Verification items for the finished model (mm, model axes). A direction names the side the tool comes from. Coordinates: 2 decimals unless noted, no trailing zeros. Write each loop counter-clockwise with the first axis right and the second up, starting at its lowest first coordinate (ties: lowest second). Pieces come first, ordered by that corner, then holes. Notation, with made-up numbers: M 10.25,69 L 24.25,69 A17 ccw 24.25,81 Z; hole C 82,51.25 d7. An arc over 180 degrees is marked long. Answer in a Markdown table with one row per item.
from build123d import *

# Parameters (mm, degrees)
BOX024_W                  = 130
BOX024_H                  = 2
BOX024_DEPTH              = 2
BOX025_W                  = 79
BOX025_H                  = 2
BOX025_DEPTH              = 2
BOX026_W                  = 2
BOX026_H                  = 52
BOX026_DEPTH              = 2
BOX023_W                  = 2
BOX023_H                  = 53
BOX023_DEPTH              = 2
BOX018_W                  = 0.5
BOX018_H                  = 2
BOX018_DEPTH              = 12
BOX019_W                  = 0.5
BOX019_H                  = 2
BOX019_DEPTH              = 12
BOX020_W                  = 0.5
BOX020_H                  = 2
BOX020_DEPTH              = 12
BOX021_W                  = 0.5
BOX021_H                  = 2
BOX021_DEPTH              = 12
BOX022_W                  = 0.5
BOX022_H                  = 2
BOX022_DEPTH              = 12
BOX017_W                  = 0.5
BOX017_H                  = 2
BOX017_DEPTH              = 12
BOX015_W                  = 12
BOX015_H                  = 10
BOX015_DEPTH              = 20
BOX016_W                  = 12
BOX016_H                  = 10
BOX016_DEPTH              = 20
BOX014_W                  = 12
BOX014_H                  = 10
BOX014_DEPTH              = 20
CYLINDER016_R             = 7
CYLINDER016_DEPTH         = 1.5
CYLINDER015_R             = 6
CYLINDER015_DEPTH         = 18
FUSION006_PLACEMENT_ANGLE = 90
CYLINDER018_R             = 7
CYLINDER018_DEPTH         = 1.5
CYLINDER017_R             = 6
CYLINDER017_DEPTH         = 18
FUSION007_PLACEMENT_ANGLE = 90
CYLINDER014_R             = 7
CYLINDER014_DEPTH         = 1.5
CYLINDER013_R             = 6
CYLINDER013_DEPTH         = 18
FUSION005_PLACEMENT_ANGLE = 90
BOX013_W                  = 33
BOX013_H                  = 77
BOX013_DEPTH              = 17
BOX012_W                  = 10
BOX012_H                  = 11
BOX012_DEPTH              = 21
BOX011_W                  = 13.5
BOX011_H                  = 11
BOX011_DEPTH              = 21
CYLINDER010_R             = 3.1
CYLINDER010_DEPTH         = 20
CYLINDER011_R             = 3.1
CYLINDER011_DEPTH         = 20
CYLINDER012_R             = 3.1
CYLINDER012_DEPTH         = 20
BOX004_W                  = 20
BOX004_H                  = 67
BOX004_DEPTH              = 20
BOX005_W                  = 20
BOX005_H                  = 67
BOX005_DEPTH              = 20
BOX006_W                  = 20
BOX006_H                  = 67
BOX006_DEPTH              = 20
BOX007_W                  = 14
BOX007_H                  = 40
BOX007_DEPTH              = 20
BOX008_W                  = 54
BOX008_H                  = 69
BOX008_DEPTH              = 20
BOX009_W                  = 30
BOX009_H                  = 52
BOX009_DEPTH              = 20
BOX010_W                  = 72
BOX010_H                  = 52
BOX010_DEPTH              = 6
CYLINDER009_R             = 3.1
CYLINDER009_DEPTH         = 20
BOX_W                     = 192
BOX_H                     = 81
BOX_DEPTH                 = 22
FILLET_R                  = 3


with BuildPart() as cube011:
    # Box024 → Box024 (new body)
    with BuildSketch(Plane(origin=(12, 75, 21), x_dir=(1, 0, 0), z_dir=(0, 0, 1))):
        with Locations((65, 1)):
            Rectangle(BOX024_W, BOX024_H)
    extrude(amount=BOX024_DEPTH)


with BuildPart() as cube012:
    # Box025 → Box025 (new body)
    with BuildSketch(Plane(origin=(12, 4, 21), x_dir=(1, 0, 0), z_dir=(0, 0, 1))):
        with Locations((39.5, 1)):
            Rectangle(BOX025_W, BOX025_H)
    extrude(amount=BOX025_DEPTH)


with BuildPart() as cube013:
    # Box026 → Box026 (new body)
    with BuildSketch(Plane(origin=(186, 14, 21), x_dir=(1, 0, 0), z_dir=(0, 0, 1))):
        with Locations((1, 26)):
            Rectangle(BOX026_W, BOX026_H)
    extrude(amount=BOX026_DEPTH)


with BuildPart() as latches:
    # Box023 → Box023 (new body)
    with BuildSketch(Plane(origin=(2, 14, 21), x_dir=(1, 0, 0), z_dir=(0, 0, 1))):
        with Locations((1, 26.5)):
            Rectangle(BOX023_W, BOX023_H)
    extrude(amount=BOX023_DEPTH)

    # Compound: union Cube011, Cube012, Cube013
    add(cube011.part)
    add(cube012.part)
    add(cube013.part)


with BuildPart() as cube005:
    # Box018 → Box018 (new body)
    with BuildSketch(Plane(origin=(163.5, 0, 9), x_dir=(1, 0, 0), z_dir=(0, 0, 1))):
        with Locations((0.25, 1)):
            Rectangle(BOX018_W, BOX018_H)
    extrude(amount=BOX018_DEPTH)


with BuildPart() as cube006:
    # Box019 → Box019 (new body)
    with BuildSketch(Plane(origin=(167.5, 0, 9), x_dir=(1, 0, 0), z_dir=(0, 0, 1))):
        with Locations((0.25, 1)):
            Rectangle(BOX019_W, BOX019_H)
    extrude(amount=BOX019_DEPTH)


with BuildPart() as cube007:
    # Box020 → Box020 (new body)
    with BuildSketch(Plane(origin=(179, 0, 9), x_dir=(1, 0, 0), z_dir=(0, 0, 1))):
        with Locations((0.25, 1)):
            Rectangle(BOX020_W, BOX020_H)
    extrude(amount=BOX020_DEPTH)


with BuildPart() as cube008:
    # Box021 → Box021 (new body)
    with BuildSketch(Plane(origin=(175.5, 79, 9), x_dir=(1, 0, 0), z_dir=(0, 0, 1))):
        with Locations((0.25, 1)):
            Rectangle(BOX021_W, BOX021_H)
    extrude(amount=BOX021_DEPTH)


with BuildPart() as cube009:
    # Box022 → Box022 (new body)
    with BuildSketch(Plane(origin=(164, 79, 9), x_dir=(1, 0, 0), z_dir=(0, 0, 1))):
        with Locations((0.25, 1)):
            Rectangle(BOX022_W, BOX022_H)
    extrude(amount=BOX022_DEPTH)


with BuildPart() as obj1:
    # Box017 → Box017 (new body)
    with BuildSketch(Plane(origin=(152, 0, 9), x_dir=(1, 0, 0), z_dir=(0, 0, 1))):
        with Locations((0.25, 1)):
            Rectangle(BOX017_W, BOX017_H)
    extrude(amount=BOX017_DEPTH)

    # Fusion010: union Cube005, Cube006, Cube007, Cube008, Cube009
    add(cube005.part)
    add(cube006.part)
    add(cube007.part)
    add(cube008.part)
    add(cube009.part)


with BuildPart() as cube002:
    # Box015 → Box015 (new body)
    with BuildSketch(Plane(origin=(167.5, 0, 13), x_dir=(1, 0, 0), z_dir=(0, 0, 1))):
        with Locations((6, 5)):
            Rectangle(BOX015_W, BOX015_H)
    extrude(amount=BOX015_DEPTH)


with BuildPart() as cube003:
    # Box016 → Box016 (new body)
    with BuildSketch(Plane(origin=(164, 71, 13), x_dir=(1, 0, 0), z_dir=(0, 0, 1))):
        with Locations((6, 5)):
            Rectangle(BOX016_W, BOX016_H)
    extrude(amount=BOX016_DEPTH)


with BuildPart() as fusion009:
    # Box014 → Box014 (new body)
    with BuildSketch(Plane(origin=(152, 0, 13), x_dir=(1, 0, 0), z_dir=(0, 0, 1))):
        with Locations((6, 5)):
            Rectangle(BOX014_W, BOX014_H)
    extrude(amount=BOX014_DEPTH)

    # Fusion009: union Cube002, Cube003
    add(cube002.part)
    add(cube003.part)


with BuildPart() as cylinder016:
    # Cylinder016 → Cylinder016 (new body)
    with BuildSketch(Plane.XY):
        Circle(CYLINDER016_R)
    extrude(amount=CYLINDER016_DEPTH)


with BuildPart() as fusion006:
    # Cylinder015 → Cylinder015 (new body)
    with BuildSketch(Plane.XY):
        Circle(CYLINDER015_R)
    extrude(amount=CYLINDER015_DEPTH)

    # Fusion006: union Cylinder016
    add(cylinder016.part)


with BuildPart() as fusion006_1:
    # Fusion006 placement: moved
    add(fusion006.part.moved(Location((158, -2, 13))).rotate(Axis((158, -2, 13), (-1, 0, 0)), FUSION006_PLACEMENT_ANGLE))


with BuildPart() as cylinder018:
    # Cylinder018 → Cylinder018 (new body)
    with BuildSketch(Plane.XY):
        Circle(CYLINDER018_R)
    extrude(amount=CYLINDER018_DEPTH)


with BuildPart() as fusion007:
    # Cylinder017 → Cylinder017 (new body)
    with BuildSketch(Plane.XY):
        Circle(CYLINDER017_R)
    extrude(amount=CYLINDER017_DEPTH)

    # Fusion007: union Cylinder018
    add(cylinder018.part)


with BuildPart() as fusion007_1:
    # Fusion007 placement: moved
    add(fusion007.part.moved(Location((170, 82.5, 13))).rotate(Axis((170, 82.5, 13), (1, 0, 0)), FUSION007_PLACEMENT_ANGLE))


with BuildPart() as cylinder014:
    # Cylinder014 → Cylinder014 (new body)
    with BuildSketch(Plane.XY):
        Circle(CYLINDER014_R)
    extrude(amount=CYLINDER014_DEPTH)


with BuildPart() as dc_jack_holes:
    # Cylinder013 → Cylinder013 (new body)
    with BuildSketch(Plane.XY):
        Circle(CYLINDER013_R)
    extrude(amount=CYLINDER013_DEPTH)

    # Fusion005: union Cylinder014
    add(cylinder014.part)


with BuildPart() as dc_jack_holes_1:
    # Fusion005 placement: moved
    add(dc_jack_holes.part.moved(Location((173.5, -2, 13))).rotate(Axis((173.5, -2, 13), (-1, 0, 0)), FUSION005_PLACEMENT_ANGLE))

    # Fusion008: union Fusion006, Fusion007
    add(fusion006_1.part)
    add(fusion007_1.part)


with BuildPart() as cube:
    # Box013 → Box013 (new body)
    with BuildSketch(Plane(origin=(149, 2, 4), x_dir=(1, 0, 0), z_dir=(0, 0, 1))):
        with Locations((16.5, 38.5)):
            Rectangle(BOX013_W, BOX013_H)
    extrude(amount=BOX013_DEPTH)


with BuildPart() as obj2:
    # Box012 → Box012 (new body)
    with BuildSketch(Plane(origin=(138.5, -1, 4), x_dir=(1, 0, 0), z_dir=(0, 0, 1))):
        with Locations((5, 5.5)):
            Rectangle(BOX012_W, BOX012_H)
    extrude(amount=BOX012_DEPTH)


with BuildPart() as arduino_jacks_holes:
    # Box011 → Box011 (new body)
    with BuildSketch(Plane(origin=(106.5, -1, 4), x_dir=(1, 0, 0), z_dir=(0, 0, 1))):
        with Locations((6.75, 5.5)):
            Rectangle(BOX011_W, BOX011_H)
    extrude(amount=BOX011_DEPTH)

    # Fusion004: union obj2
    add(obj2.part)


with BuildPart() as m4_mounting_hole001:
    # Cylinder010 → Cylinder010 (new body)
    with BuildSketch(Plane(origin=(2, 77, 1), x_dir=(1, 0, 0), z_dir=(0, 0, 1))):
        Circle(CYLINDER010_R)
    extrude(amount=CYLINDER010_DEPTH)


with BuildPart() as m4_mounting_hole002:
    # Cylinder011 → Cylinder011 (new body)
    with BuildSketch(Plane(origin=(186, 77, 1), x_dir=(1, 0, 0), z_dir=(0, 0, 1))):
        Circle(CYLINDER011_R)
    extrude(amount=CYLINDER011_DEPTH)


with BuildPart() as m4_mounting_hole003:
    # Cylinder012 → Cylinder012 (new body)
    with BuildSketch(Plane(origin=(186, 4, 1), x_dir=(1, 0, 0), z_dir=(0, 0, 1))):
        Circle(CYLINDER012_R)
    extrude(amount=CYLINDER012_DEPTH)


with BuildPart() as obj3:
    # Box004 → Box004 (new body)
    with BuildSketch(Plane(origin=(6, 7, 1), x_dir=(1, 0, 0), z_dir=(0, 0, 1))):
        with Locations((10, 33.5)):
            Rectangle(BOX004_W, BOX004_H)
    extrude(amount=BOX004_DEPTH)


with BuildPart() as obj4:
    # Box005 → Box005 (new body)
    with BuildSketch(Plane(origin=(29, 7, 1), x_dir=(1, 0, 0), z_dir=(0, 0, 1))):
        with Locations((10, 33.5)):
            Rectangle(BOX005_W, BOX005_H)
    extrude(amount=BOX005_DEPTH)


with BuildPart() as obj5:
    # Box006 → Box006 (new body)
    with BuildSketch(Plane(origin=(52, 7, 1), x_dir=(1, 0, 0), z_dir=(0, 0, 1))):
        with Locations((10, 33.5)):
            Rectangle(BOX006_W, BOX006_H)
    extrude(amount=BOX006_DEPTH)


with BuildPart() as obj6:
    # Box007 → Box007 (new body)
    with BuildSketch(Plane(origin=(74, 18, 1), x_dir=(1, 0, 0), z_dir=(0, 0, 1))):
        with Locations((7, 20)):
            Rectangle(BOX007_W, BOX007_H)
    extrude(amount=BOX007_DEPTH)


with BuildPart() as obj7:
    # Box008 → Box008 (new body)
    with BuildSketch(Plane(origin=(98, 2, 1), x_dir=(1, 0, 0), z_dir=(0, 0, 1))):
        with Locations((27, 34.5)):
            Rectangle(BOX008_W, BOX008_H)
    extrude(amount=BOX008_DEPTH)


with BuildPart() as obj8:
    # Box009 → Box009 (new body)
    with BuildSketch(Plane(origin=(156, 14, 1), x_dir=(1, 0, 0), z_dir=(0, 0, 1))):
        with Locations((15, 26)):
            Rectangle(BOX009_W, BOX009_H)
    extrude(amount=BOX009_DEPTH)


with BuildPart() as obj9:
    # Box010 → Box010 (new body)
    with BuildSketch(Plane(origin=(89, 19, 15), x_dir=(1, 0, 0), z_dir=(0, 0, 1))):
        with Locations((36, 26)):
            Rectangle(BOX010_W, BOX010_H)
    extrude(amount=BOX010_DEPTH)


with BuildPart() as obj10:
    # Cylinder009 → Cylinder009 (new body)
    with BuildSketch(Plane(origin=(2, 4, 1), x_dir=(1, 0, 0), z_dir=(0, 0, 1))):
        Circle(CYLINDER009_R)
    extrude(amount=CYLINDER009_DEPTH)

    # Fusion003: union M4 Mounting Hole001, M4 Mounting Hole002, M4 Mounting Hole003, obj3, obj4, obj5, obj6, obj7, obj8, obj9
    add(m4_mounting_hole001.part)
    add(m4_mounting_hole002.part)
    add(m4_mounting_hole003.part)
    add(obj3.part)
    add(obj4.part)
    add(obj5.part)
    add(obj6.part)
    add(obj7.part)
    add(obj8.part)
    add(obj9.part)


with BuildPart() as body:
    # Box → Box (new body)
    with BuildSketch(Plane(origin=(-2, 0, -1), x_dir=(1, 0, 0), z_dir=(0, 0, 1))):
        with Locations((96, 40.5)):
            Rectangle(BOX_W, BOX_H)
    extrude(amount=BOX_DEPTH)

    # Cut: cut obj10
    add(obj10.part, mode=Mode.SUBTRACT)

    # Cut001: cut Arduino Jacks Holes
    add(arduino_jacks_holes.part, mode=Mode.SUBTRACT)

    # Cut002: cut Cube
    add(cube.part, mode=Mode.SUBTRACT)

    # Cut003: cut DC_Jack_Holes
    add(dc_jack_holes_1.part, mode=Mode.SUBTRACT)

    # Cut004: cut Fusion009
    add(fusion009.part, mode=Mode.SUBTRACT)

    # Fillet
    fillet_edges = [body.edges().sort_by_distance(p)[0] for p in [
        (-2, 0, 10),
        (-2, 81, 10),
        (190, 0, 10),
        (190, 81, 10),
    ]]
    fillet(fillet_edges, radius=FILLET_R)

    # Fusion011: union obj1
    add(obj1.part)

    # Fusion012: union Latches
    add(latches.part)


solid = body.part
1) Sectioned sample at A-A (z = 19). Give the number of separate pieces and of enclosed holes in the cut face, then the cut area to 3 significant figures.
Response values:
| item | result |
|---|---|
| separate pieces | 5 |
| enclosed holes | 8 |
| area | 3,990 mm² |
2) Depth check by flat-ended pin: pin 1 (22 mm diameter, centred on x = 43, y = 41, fed in from +Z); pin 2 (1.5 mm diameter, centred on x = 63, y = 14.5, fed in from +Z); pin 3 (0.6 mm diameter, centred on x = 35.5, z = 22.5, fed in from +Y). Enter the tip coordinate at first touch or a pass-through.
Response values:
| item | result |
|---|---|
| pin 1 | stops at z = 21 |
| pin 2 | stops at z = 1 |
| pin 3 | stops at y = 77 |
3) Thickness scan on L1, parallel to X at y = 10, z = 11.25; L2, parallel to Y at x = 2, z = 8.75; L3, parallel to X at y = 31, z = 10.75. Record the ranges inside material, lowest first. Write a range as [from, to].
Response values:
| item | result |
|---|---|
| L1 | x = [-2, 6], [26, 29], [49, 52], [72, 98], [182, 190] |
| L2 | y = [0, 0.9], [7.1, 73.9], [80.1, 81] |
| L3 | x = [-2, 6], [26, 29], [49, 52], [72, 74], [88, 98], [186, 190] |
4) Sectioned sample at C-C (y = 9.5). Record the cut outline in (x, z), then the cut area to 3 significant figures.
Response values:
| item | result |
|---|---|
| outline | M -2,-1 L 190,-1 L 190,21 L 182,21 L 182,4 L 152,4 L 152,1 L 98,1 L 98,21 L 72,21 L 72,1 L 52,1 L 52,21 L 49,21 L 49,1 L 29,1 L 29,21 L 26,21 L 26,1 L 6,1 L 6,21 L -2,21 Z |
| area | 1,430 mm² |
5) Sectioned sample at D-D (x = 85.5). Record the cut outline in (y, z), then the cut area to 3 significant figures.
Response values:
| item | result |
|---|---|
| outline | M 0,-1 L 81,-1 L 81,21 L 77,21 L 77,23 L 75,23 L 75,21 L 58,21 L 58,1 L 18,1 L 18,21 L 6,21 L 6,23 L 4,23 L 4,21 L 0,21 Z |
| area | 990 mm² |
6) Tool access check on faces 1 (the face through (74, 38, 11)), 2 (the face through (170, 80, 7)). Record the directions out of +Z, -Z, +X, -X, +Y, -Y that give a thin tool (end or side, any length) a straight path to the whole face; none if there is none.
Response values:
| item | result |
|---|---|
| face 1 | +Z |
| face 2 | +Z, +Y |
7) Release check for a two-part mould opening along X. For faces 3 (the face through (93, 81, 10)), 4 (the face through (190, 40, 10)), 5 (the face through (16, 41, 1)) record: +X half, -X half, draft (parallel to the pull), parting line (faces both ways), or undercut.
Response values:
| item | result |
|---|---|
| face 3 | draft |
| face 4 | +X half |
| face 5 | undercut |
8) Sectioned sample at B-B (x = 14.5). Record the cut outline in (y, z).
Response values:
| item | result |
|---|---|
| outline | M 0,-1 L 81,-1 L 81,21 L 77,21 L 77,23 L 75,23 L 75,21 L 74,21 L 74,1 L 7,1 L 7,21 L 6,21 L 6,23 L 4,23 L 4,21 L 0,21 Z |
